The model under review builds one solid part; all positions refer to its coordinate system, in mm. A direction names the side the tool comes from. Give positions to 0.01 mm unless a question says otherwise; leave off trailing zeros. Loops run counter-clockwise (first coordinate to the right, second up) from the corner with the lowest first, then second, coordinate; pieces in that order, holes last. Notation, with made-up numbers: M 68.5,4.25 L 91.5,4.25 A13 cw 91.5,22.25 Z; hole C -7,-35 d8. An arc over 180 degrees is marked long. One line per item, written item: value. Start each with the question number.
Q1. We need section C-C on y = -2.5. Write out the cut boundary in (x, z).
Q2. To check wall thickness, follow line 1 along X through (y, z) = (-2, -18.5); line 2 along Z through (x, y) = (-27, -4.75); line 3 along X through (y, z) = (-2.5, -47.5). State the ranges of each line that lie inside material, in increasing order. Write a range as from..to.
Q3. We need section B-B on z = 42. Write out the cut boundary in (x, y).
Q4. For faces 1 (the face through (45, -5, 3)), 2 (the face through (100, -5, 1)), list the 3-axis set-ups (+Z, -Z, +X, -X, +Y, -Y) from which the entire face can be reached by the end or side of a thin tool; tool diameter is ignored.
Q5. We need section A-A on x = -38. Write out the cut boundary in (y, z), plus the area to 3 significant figures.
Q6. Mouldability with a two-part tool opening along X and no side actions: class faces 3 (the face through (-1, -5, 100)), 4 (the face through (-50, -5, 1)), 5 (the face through (-100, -5, 1)), 6 (the face through (50, -5, -1)) as released by +X, released by -X, zero draft, split by the parting line, or undercut.
```python
from build123d import *

# Parameters (mm, degrees)
SKETCH_1_W          = 200
SKETCH_1_H          = 200
EXTRUDE_1_DEPTH     = 10
CUT_EXTRUDE_1_DEPTH = 10


with BuildPart() as part:
    # 草圖1 → 填料-伸長1 (new body)
    with BuildSketch(Plane(origin=(0, 0, 0), x_dir=(1, 0, 0), z_dir=(0, 1, 0))):
        Rectangle(SKETCH_1_W, SKETCH_1_H)
    extrude(amount=-EXTRUDE_1_DEPTH)

    # 草圖1<3> → 除料-伸長-薄件1 (cut)
    with BuildSketch(Plane(origin=(0, 0, 0), x_dir=(1, 0, 0), z_dir=(0, 1, 0))):
        Polygon((-50, -50), (-50, 50), (50, 50), (50, -50), (45, -50), (45, 45), (-45, 45), (-45, -50), align=None)
    extrude(amount=-CUT_EXTRUDE_1_DEPTH, mode=Mode.SUBTRACT)


solid = part.part
```
Solved:
1. outline: M -100,-100 L 100,-100 L 100,100 L -100,100 Z; hole M -50,-50 L 50,-50 L 50,50 L 45,50 L 45,-45 L -45,-45 L -45,50 L -50,50 Z
2. line 1: -100..-50, -45..45, 50..100
2. line 2: -100..-50, -45..100
2. line 3: -100..-50, 50..100
3. outline: M -100,-10 L -50,-10 L -50,0 L -100,0 Z; M -45,-10 L 45,-10 L 45,0 L -45,0 Z; M 50,-10 L 100,-10 L 100,0 L 50,0 Z
4. face 1: +Y, -Y
4. face 2: +Z, -Z, +X, +Y, -Y
5. outline: M -10,-100 L 0,-100 L 0,-50 L -10,-50 Z; M -10,-45 L 0,-45 L 0,100 L -10,100 Z
5. area: 1,950 mm2
6. face 3: zero draft
6. face 4: undercut
6. face 5: released by -X
6. face 6: undercut
